```python
from build123d import *

# Parameters (mm, degrees)
F0_W     = 32.5
F0_H     = 22
F1_DEPTH = 6.7
F2_R     = 7.5
F3_DEPTH = 13


with BuildPart() as f1:
    # F0 (on Top) → F1 (new body)
    with BuildSketch(Plane.XY):
        with Locations((1, -1)):
            Rectangle(F0_W, F0_H)
        Polygon((-8.5, 17), (-15.25, 10), (17.25, 10), (8.5, 17), align=None)
    extrude(amount=F1_DEPTH)

    # F2 (on Top) → F3 (join)
    with BuildSketch(Plane.XY):
        Circle(F2_R)
    extrude(amount=F3_DEPTH)


solid = f1.part
```
Model file for the job. Use its own axes, mm. A direction names the side the tool comes from. Coordinates: 2 decimals unless noted, no trailing zeros. Loops run counter-clockwise (first coordinate to the right, second up) from the corner with the lowest first, then second, coordinate; pieces in that order, holes last. Notation, with made-up numbers: (-38.75, 76.25) - (-23.75, 76.25) arc R16 ccw to (-23.75, 99.25) - close; hole circle Ø4 at (-2, 17). An arc over 180 degrees is marked (long way). Write item = value, one per line. Start each with the question number.
Item 1: Saw through at D-D, the plane z = 8.5. List the corners of the cut face in (x, y).
Item 2: Saw through at A-A, the plane x = 0. List the corners of the cut face in (y, z), then the cut area to 3 significant figures.
Item 3: Saw through at C-C, the plane y = 4.5. List the corners of the cut face in (x, z).
Item 4: Drop flat-ended pins along their axis: pin 1 Ø5 at (x, z) = (14, 3) entering from +Y; pin 2 Ø10 at (x, y) = (-6.5, -8) entering from -Z. Give the stop position or say it passes through.
Item 5: Saw through at B-B, the plane z = 4.5. List the corners of the cut face in (x, y), then the cut area to 3 significant figures.
Item 6: 3-axis set-ups, long thin cutter, end or side, ignore diameter. For faces 1 (the face through (-7.493, 0.33, 9.806)), 2 (the face through (1, 3, 0)): which of +Z, -Z, +X, -X, +Y, -Y reach the whole face in a straight line?
Item 7: Wall check: probe 1 along Z at (x, y) = (-12.5, 9.5); probe 2 along X at (y, z) = (-1.75, 10.5); probe 3 along Y at (x, z) = (6.5, 9.75). Give the ranges that are in metal, low to high. Write a range as [from, to].
Answers:
q1.outline = circle Ø15 at (0, 0)
q2.outline = (-12, 0) - (17, 0) - (17, 6.7) - (7.5, 6.7) - (7.5, 13) - (-7.5, 13) - (-7.5, 6.7) - (-12, 6.7) - close
q2.area = 289 mm2
q3.outline = (-15.25, 0) - (17.25, 0) - (17.25, 6.7) - (6, 6.7) - (6, 13) - (-6, 13) - (-6, 6.7) - (-15.25, 6.7) - close
q4.pin_1 = 14.6
q4.pin_2 = 0
q5.outline = (-15.25, -12) - (17.25, -12) - (17.25, 10) - (8.5, 17) - (-8.5, 17) - (-15.25, 10) - close
q5.area = 888 mm2
q6.face_1 = +Z
q6.face_2 = -Z, +X, -X, +Y, -Y
q7.probe_1 = [0, 6.7]
q7.probe_2 = [-7.29, 7.29]
q7.probe_3 = [-3.74, 3.74]
